Autodesk Fusion 360 part; units mm, degrees
sketch "Sketch1" plane through (0, 0, 0) normal (0, 0, 1) x (1, 0, 0)
  line L0 (12, 6.25) -> (-12, 6.25)
  line L1 (-12, 6.25) -> (-12, -6.25)
  line L2 (-12, -6.25) -> (12, -6.25)
  line L3 (12, -6.25) -> (12, 6.25)
  line L4 (12, 6.25) -> (-12, -6.25) construction
  line L5 (-12, 6.25) -> (12, -6.25) construction
  line L6 (12, 6.25) -> (17, 6.25)
  line L7 (17, 6.25) -> (17, -6.25)
  line L8 (12, -6.25) -> (17, -6.25)
  line L9 (-12, 6.25) -> (-17, 6.25)
  line L10 (-17, 6.25) -> (-17, -6.25)
  line L11 (-17, -6.25) -> (-12, -6.25)
  dimension "d1" = 24
  dimension "d2" = 12.5
  dimension "d3" = 5
  dimension "d4" = 5
extrude "Extrude1" add sketch "Sketch1" along normal blind 24 contours L0 L1 L2 L3
sketch "Sketch2" plane through (0, -6.25, 0) normal (0, -1, 0) x (1, 0, 0)
  line L0 (-12, 0) -> (12, 0)
  line L1 (12, 0) -> (12, 24)
  line L2 (12, 24) -> (-12, 24)
  line L3 (-12, 24) -> (-12, 0)
  line L4 (12, 24) -> (12, 23)
  line L5 (12, 23) -> (17, 23)
  line L6 (17, 23) -> (17, 20)
  line L7 (17, 20) -> (12, 20)
  line L8 (-12, 24) -> (-12, 23)
  line L9 (-12, 23) -> (-17, 23)
  line L10 (-17, 23) -> (-17, 20)
  line L11 (-17, 20) -> (-12, 20)
  dimension "d7" = 1
  dimension "d8" = 5
  dimension "d9" = 3
  dimension "d10" = 1
  dimension "d11" = 5
  dimension "d12" = 3
extrude "Extrude2" add sketch "Sketch2" against normal up to surface (12.5 mm away) contours L3 L9 L10 L11 | L1 L5 L6 L7
sketch "Sketch3" plane through (0, 0, 24) normal (0, 0, 1) x (-1, 0, 0)
  line L0 (-12, 6.25) -> (-12, -6.25)
  line L1 (-12, -6.25) -> (12, -6.25)
  line L2 (12, -6.25) -> (12, 6.25)
  line L3 (12, 6.25) -> (-12, 6.25)
  circle A0 centre (-6, 0) radius 6
  circle A1 centre (0.5, 0) radius 2.5
  dimension "d15" = 12
  dimension "d16" = 5
  dimension "d17" = 6.5
extrude "Extrude3" add sketch "Sketch3" along normal blind 6 contours A0 A1 | A0 A1 | A0 A1
sketch "Sketch4" plane through (0, 0, 30) normal (0, 0, 1) x (-1, 0, 0)
  arc A0 (-0.4615, -2.3077) -> (-0.4615, 2.3077) centre (0.5, 0) ccw
  arc A1 (-0.4615, 2.3077) -> (-0.4615, -2.3077) centre (-6, 0) ccw
  circle A2 centre (-6, 0) radius 2.5
  dimension "d20" = 5
extrude "Extrude4" add sketch "Sketch4" along normal blind 4 contours A2
sketch "Sketch5" plane through (0, 0, 23) normal (0, 0, 1) x (-1, 0, 0)
  line L0 (-17, -6.25) -> (-12, -6.25)
  line L1 (-12, -6.25) -> (-12, 6.25)
  line L2 (-12, 6.25) -> (-17, 6.25)
  line L3 (-17, 6.25) -> (-17, -6.25)
  circle A0 centre (-14.5, 0) radius 1.25
  dimension "d23" = 2.5
  dimension "d24" = 2.5
sketch "Sketch6" plane through (0, 0, 23) normal (0, 0, 1) x (-1, 0, 0)
  line L0 (12, -6.25) -> (17, -6.25)
  line L1 (17, -6.25) -> (17, 6.25)
  line L2 (17, 6.25) -> (12, 6.25)
  line L3 (12, 6.25) -> (12, -6.25)
  circle A0 centre (14.5, 0) radius 1.25
  dimension "d25" = 2.5
  dimension "d26" = 2.5
extrude "Extrude5" cut sketch "Sketch6" sketch "Sketch5" against normal blind 3 contours A0 of sketch 2 contours A0
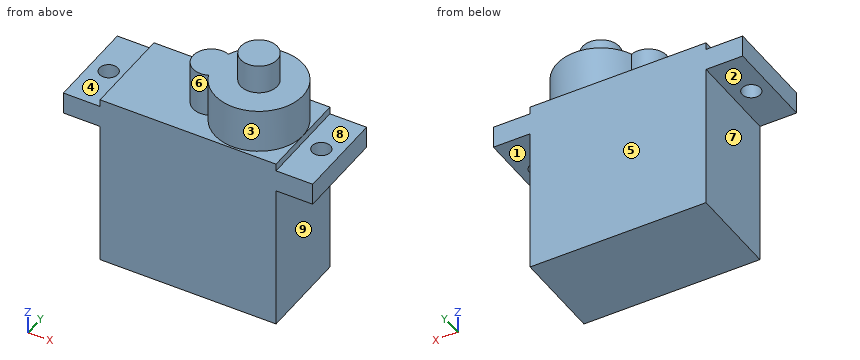
Could you check a few things on this model? Use its own coordinates, in mm. Face numbers are marked on the shaded views. A direction names the side the tool comes from. Coordinates: 2 decimals unless noted, no trailing zeros. Order: outer loops, then holes, each group sorted by start corner. A loop starts at its lowest first (then second) coordinate and runs counter-clockwise, first axis right, second up. Notation, with made-up numbers: (50, 49.25) -> (81, 49.25) arc R27 cw to (81, 70.25) -> close; hole circle Ø3 at (9, 0.25). An arc over 180 degrees is marked (long way). One line per item, written item: value. Start each with the question number.
1) Imagine slicing it at B-B on x = -2.5. List the corners of the cut face in (y, z) for me.
2) Imagine slicing it at D-D on z = 18. List the corners of the cut face in (x, y) for me.
3) If I drill on L1, parallel to X at y = 0, z = 22.15; L2, parallel to Y at x = -14.5, z = 21.3; L3, parallel to X at y = -0.5, z = 11.5, over which ranges is the centre line in solid material (lowest first)? Write a range as [from, to].
4) Imagine slicing it at C-C on y = 3.5. List the corners of the cut face in (x, z) for me.
5) I'm going to push flat-ended pins straight in: pin 1 (0.8 mm diameter, centred on y = -2.5, z = 23.5, fed in from -X); pin 2 (4 mm diameter, centred on x = 14.5, y = 0.5, fed in from +Z); pin 3 (2.5 mm diameter, centred on x = -15, y = 2.5, fed in from -Z). Where does each tip first touch, or does it pass through?
6) Imagine slicing it at A-A on x = 14.5. List the corners of the cut face in (y, z) for me, plus the area to 3 significant figures.
7) We'd pull the mould along X, two halves only. Please class the marked faces 6, 7, 8 and 9: +X half, -X half, draft (parallel to the pull), parting line (faces both ways), or undercut.
8) Which directions (+Z, -Z, +X, -X, +Y, -Y) give clear straight access to the entire face, cutting with the end or side of a thin tool? Please do the marked faces 1, 2, 3, 4 and 5.
Answer list:
1. outline: (-6.25, 0) -> (6.25, 0) -> (6.25, 24) -> (1.5, 24) -> (1.5, 30) -> (-1.5, 30) -> (-1.5, 24) -> (-6.25, 24) -> close
2. outline: (-12, -6.25) -> (12, -6.25) -> (12, 6.25) -> (-12, 6.25) -> close
3. L1: x = [-17, -15.75], [-13.25, 13.25], [15.75, 17]
3. L2: y = [-6.25, -1.25], [1.25, 6.25]
3. L3: x = [-12, 12]
4. outline: (-17, 20) -> (-12, 20) -> (-12, 0) -> (12, 0) -> (12, 20) -> (17, 20) -> (17, 23) -> (12, 23) -> (12, 24) -> (10.87, 24) -> (10.87, 30) -> (1.13, 30) -> (1.13, 24) -> (-12, 24) -> (-12, 23) -> (-17, 23) -> close
5. pin 1: stops at x = -12
5. pin 2: stops at z = 23
5. pin 3: stops at z = 20
6. outline: (-6.25, 20) -> (-1.25, 20) -> (-1.25, 23) -> (-6.25, 23) -> close; (1.25, 20) -> (6.25, 20) -> (6.25, 23) -> (1.25, 23) -> close
6. area: 30.0 mm2
7. face 6: undercut
7. face 7: -X half
7. face 8: draft
7. face 9: +X half
8. face 1: -Z, +X, +Y, -Y
8. face 2: -Z, -X, +Y, -Y
8. face 3: +Z
8. face 4: +Z, -X, +Y, -Y
8. face 5: +Z, -Z, +X, -X, +Y
